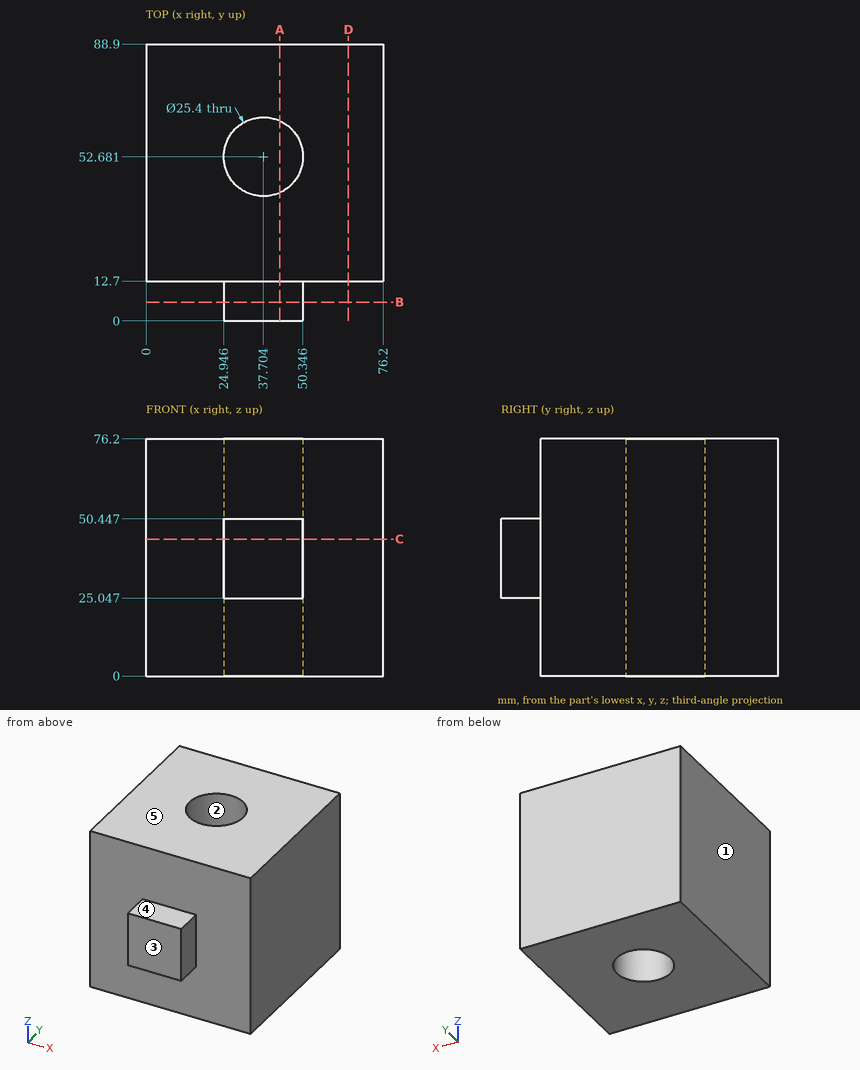
Here's the drawing with two shaded views (mm, measured from the low corner). I have some questions. A direction names the side the tool comes from. Round coordinates to 2 decimals unless told otherwise and drop trailing zeros. Loops run counter-clockwise (first coordinate to the right, second up) from the corner with the lowest first, then second, coordinate; pieces in that order, holes last. Notation, with made-up numbers: (59.25, -1) -> (88.25, -1) arc R24 cw to (88.25, 16) -> close; hole circle Ø8 at (39.25, 76.5). An arc over 180 degrees is marked (long way). Answer as CSV lines item,"result". Start each with the question number.
1. Imagine slicing it at A-A on x = 43. Write out the boundary of the cut face in (y, z).
2. Imagine slicing it at D-D on x = 65. Write out the boundary of the cut face in (y, z).
3. I need wall thicknesses on probe 1 along Y at (x, z) = (8, 70.5); probe 2 along X at (y, z) = (59, 36); probe 3 along Z at (x, y) = (32, 8.5). Which ranges of each line are inside material? Lowest first, please. Write a range as from..to.
4. For the marked faces 4 and 5, which set-ups out of +Z, -Z, +X, -X, +Y, -Y let a thin tool reach every point of the face, with its end or its side?
5. I'm going to push flat-ended pins straight in: P1, Ø6.5, axis at y = 3, z = 35, coming from the +X side; P2, Ø4, axis at x = 36, y = 8, coming from the +Z side; P3, Ø10, axis at x = 43.5, y = 7, coming from the -Z side. Where does each tip first touch, or does it pass through?
6. If we mould it in two halves opening along X, with no side actions, what happens to the marked faces 1, 2 and 3? For each: pulls with the +X half, pulls with the -X half, needs draft (parallel to the pull), parting line crosses it, or undercut.
7. Imagine slicing it at C-C on z = 44. Write out the boundary of the cut face in (x, y).
8. Imagine slicing it at B-B on y = 6. Write out the boundary of the cut face in (x, z).
Solution:
1,outline,"(0, 25.05) -> (12.7, 25.05) -> (12.7, 0) -> (41.14, 0) -> (41.14, 76.2) -> (12.7, 76.2) -> (12.7, 50.45) -> (0, 50.45) -> close; (64.22, 0) -> (88.9, 0) -> (88.9, 76.2) -> (64.22, 76.2) -> close"
2,outline,"(12.7, 0) -> (88.9, 0) -> (88.9, 76.2) -> (12.7, 76.2) -> close"
3,probe 1,"12.7..88.9"
3,probe 2,"0..26.69, 48.72..76.2"
3,probe 3,"25.05..50.45"
4,face 4,"+Z, +X, -X, -Y"
4,face 5,"+Z, +X, -X, +Y, -Y"
5,P1,"x = 50.35"
5,P2,"z = 50.45"
5,P3,"z = 25.05"
6,face 1,"pulls with the -X half"
6,face 2,"undercut"
6,face 3,"needs draft"
7,outline,"(0, 12.7) -> (24.95, 12.7) -> (24.95, 0) -> (50.35, 0) -> (50.35, 12.7) -> (76.2, 12.7) -> (76.2, 88.9) -> (0, 88.9) -> close; hole circle Ø25.4 at (37.7, 52.68)"
8,outline,"(24.95, 25.05) -> (50.35, 25.05) -> (50.35, 50.45) -> (24.95, 50.45) -> close"
